from build123d import *

# Parameters (mm, degrees)
F0_R     = 408.94
F0_R_2   = 185.801
F1_DEPTH = 749.3
F0_R_3   = 762
F0_R_4   = 63.5
F2_DEPTH = 378.46
F3_R     = 81.28
F4_R     = 81.28


with BuildPart() as f1:
    # F0 (on Top) → F1 (new body)
    with BuildSketch(Plane.XY):
        Circle(F0_R)
        Circle(F0_R_2, mode=Mode.SUBTRACT)
    extrude(amount=F1_DEPTH)

    # F0 (on Top) → F2 (join)
    with BuildSketch(Plane.XY):
        Circle(F0_R_3)
        with Locations((0, -566.42)):
            Circle(F0_R_4, mode=Mode.SUBTRACT)
        with Locations((-566.42, 0)):
            Circle(F0_R_4, mode=Mode.SUBTRACT)
        Circle(F0_R, mode=Mode.SUBTRACT)
        with Locations((566.42, 0)):
            Circle(F0_R_4, mode=Mode.SUBTRACT)
        with Locations((0, 566.42)):
            Circle(F0_R_4, mode=Mode.SUBTRACT)
    extrude(amount=F2_DEPTH)

    # F3
    f3_edges = [f1.edges().sort_by_distance(p)[0] for p in [
        (-408.94, 0, 749.3),
    ]]
    fillet(f3_edges, radius=F3_R)

    # F4
    f4_edges = [f1.edges().sort_by_distance(p)[0] for p in [
        (-762, 0, 378.46),
    ]]
    fillet(f4_edges, radius=F4_R)


solid = f1.part
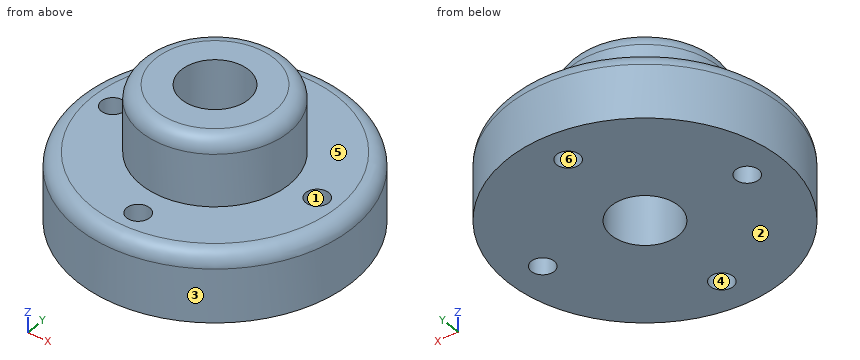
Build history of the part. All positions in model axes, mm. Face numbers are marked on the shaded views. A direction names the side the tool comes from. Give positions to 0.01 mm unless a question says otherwise; leave off trailing zeros. Write each loop counter-clockwise with the first axis right and the second up, starting at its lowest first coordinate (ties: lowest second). Pieces come first, ordered by that corner, then holes. Notation, with made-up numbers: (21, 2.25) - (75, 2.25) arc R18 ccw to (75, 28.25) - close; hole circle Ø10 at (-34, 8.5). An arc over 180 degrees is marked (long way). Use one line per item in the form item = value. Start each with the question number.
1. 3-axis set-ups, long thin cutter, end or side, ignore diameter. For the marked faces 5 and 6: which of +Z, -Z, +X, -X, +Y, -Y reach the whole face in a straight line?
2. Band-saw the part on A-A on x = 0. Write the cut outline in (y, z).
3. Probe line 1 (Z direction, x = 390, y = -518.5); line 2 (Y direction, x = 37.5, z = 666); line 3 (Y direction, x = 29, z = 405). List the from-to ranges inside material, lowest first. Write a range as [from, to].
4. Drop flat-ended pins along their axis: pin 1 Ø1 at (x, y) = (-20.5, -507.5) entering from +Z; pin 2 Ø5 at (x, z) = (114.5, 594.5) entering from -Y; pin 3 Ø5 at (x, y) = (354.5, -498) entering from +Z; pin 4 Ø5 at (x, z) = (-243, 476) entering from +Y. Give the stop position or say it passes through.
5. Two-plate mould, pull along Y, no slides. Class the marked faces 1, 2, 3 and 4: released by +Y, released by -Y, zero draft, split by the parting line, or undercut.
6. Band-saw the part on C-C on z = 508. Write the cut outline in (x, y), plus the area to 3 significant figures.
7. Band-saw the part on D-D on z = 120. Write the cut outline in (x, y).
Conclusion:
q1.face_5 = +Z
q1.face_6 = +Z, -Z
q2.outline = (-762, 0) - (-629.92, 0) - (-629.92, 378.46) - (-680.72, 378.46) arc R81.28 ccw to (-762, 297.18) - close; (-502.92, 0) - (-185.8, 0) - (-185.8, 749.3) - (-327.66, 749.3) arc R81.28 ccw to (-408.94, 668.02) - (-408.94, 378.46) - (-502.92, 378.46) - close; (185.8, 0) - (502.92, 0) - (502.92, 378.46) - (408.94, 378.46) - (408.94, 668.02) arc R81.28 ccw to (327.66, 749.3) - (185.8, 749.3) - close; (629.92, 0) - (762, 0) - (762, 297.18) arc R81.28 ccw to (680.72, 378.46) - (629.92, 378.46) - close
q3.line_1 = [0, 378.46]
q3.line_2 = [-407.22, -181.98], [181.98, 407.22]
q3.line_3 = [-407.91, -183.52], [183.52, 407.91]
q4.pin_1 = through
q4.pin_2 = -393.3
q4.pin_3 = 378.46
q4.pin_4 = 330.74
q5.face_1 = undercut
q5.face_2 = zero draft
q5.face_3 = split by the parting line
q5.face_4 = undercut
q6.outline = circle Ø817.88 at (0, 0); hole circle Ø371.6 at (0, 0)
q6.area = 417,000 mm²
q7.outline = circle Ø1524 at (0, 0); hole circle Ø127 at (-566.42, 0); hole circle Ø371.6 at (0, 0); hole circle Ø127 at (0, -566.42); hole circle Ø127 at (0, 566.42); hole circle Ø127 at (566.42, 0)
